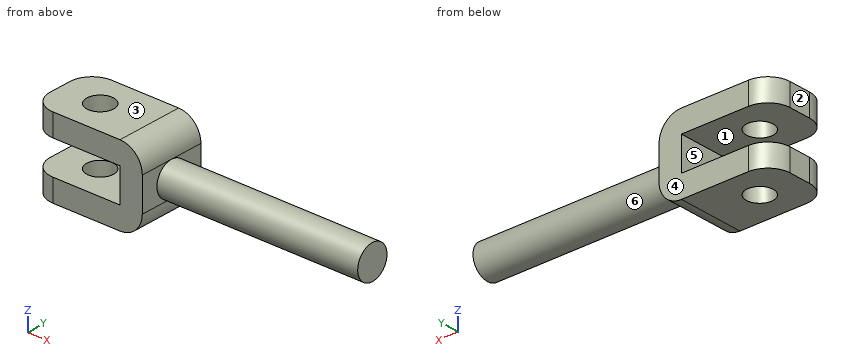
```python
from build123d import *

# Parameters (mm, degrees)
SKETCH1_R                = 0.75
BOSS_EXTRUDE1_DEPTH      = 10
BOSS_EXTRUDE2_DEPTH      = 1.5
BOSS_EXTRUDE2_DEPTH_BACK = 1.5
FILLET1_R                = 1
SKETCH3_R                = 0.6
CUT_EXTRUDE1_DEPTH       = 5


with BuildPart() as part:
    # Sketch1 → Boss-Extrude1 (new body)
    with BuildSketch(Plane(origin=(0, 0, 0), x_dir=(0, 0, -1), z_dir=(1, 0, 0))):
        Circle(SKETCH1_R)
    extrude(amount=BOSS_EXTRUDE1_DEPTH)

    # Sketch2 → Boss-Extrude2 (add, two sides: drawn at the far end of the back side and taken through both)
    with BuildSketch(Plane(origin=(0, 0, 0), x_dir=(1, 0, 0), z_dir=(0, 1, 0)).offset(-BOSS_EXTRUDE2_DEPTH_BACK)):
        Polygon((1, 1.75), (1, -1.75), (-4, -1.75), (-4, -0.75), (0, -0.75), (0, 0.75), (-4, 0.75), (-4, 1.75), align=None)
    extrude(amount=BOSS_EXTRUDE2_DEPTH + BOSS_EXTRUDE2_DEPTH_BACK)

    # Fillet1
    fillet1_edges = [part.edges().sort_by_distance(p)[0] for p in [
        (-4, 1.5, 1.25),
        (-4, 1.5, -1.25),
        (-4, -1.5, -1.25),
        (1, 0, -1.75),
        (1, 0, 1.75),
        (-4, -1.5, 1.25),
    ]]
    fillet(fillet1_edges, radius=FILLET1_R - 0.0001)  # a hair under: the kernel refuses the full size

    # Sketch3 → Cut-Extrude1 (cut)
    with BuildSketch(Plane(origin=(0, 0, -1.75), x_dir=(-1, 0, 0), z_dir=(0, 0, -1))):
        with Locations((2.2, 0)):
            Circle(SKETCH3_R)
    extrude(amount=-CUT_EXTRUDE1_DEPTH, mode=Mode.SUBTRACT)


solid = part.part
```
Geometry check sheet. Reference: the model listing, model coordinates, mm. Face numbers are marked on the shaded views. A direction names the side the tool comes from. Coordinates: 2 decimals unless noted, no trailing zeros. Order: outer loops, then holes, each group sorted by start corner. A loop starts at its lowest first (then second) coordinate and runs counter-clockwise, first axis right, second up. Notation, with made-up numbers: M 50,87.5 L 94,87.5 A12 ccw 94,107.5 Z; hole C -39,12 d6. An arc over 180 degrees is marked long. One line per question, with ' | ' between items. Start each with the question number.
Item 1: Gauge pin test, flat ends, axial feed: pin 1 (0.8 mm diameter, centred on y = 0.5, z = 0, fed in from -X); pin 2 (1.5 mm diameter, centred on x = 2, y = -1, fed in from +Z). Record the tip position at first contact, or that the pin passes through.
Item 2: Cross-section at B-B on z = 0. Enter the section's corners in (x, y), then the cut area to 3 significant figures.
Item 3: Cross-section at A-A on x = -2.2. Enter the section's corners in (y, z).
Item 4: Set-up check for the marked faces 4, 5 and 6: record each of +Z, -Z, +X, -X, +Y, -Y from which the full face is reachable in a straight line by a thin tool's end or side.
Item 5: Draft check along Z on the marked faces 1, 2 and 3. Enter one of: pulls with the +Z half, pulls with the -Z half, needs draft (parallel to the pull), parting line crosses it, or undercut.
Item 6: Cross-section at D-D on x = 8. Enter the section's corners in (y, z), then the cut area to 3 significant figures.
Item 7: Material ranges on L1, parallel to Z at x = -0.5, y = -0.2; L2, parallel to Y at x = -2.2, z = -1.15; L3, parallel to X at y = 0.75, z = 0.55, recorded low to high. Write a range as [from, to].
Item 8: Cross-section at C-C on z = -1. Enter the section's corners in (x, y), then the cut area to 3 significant figures.
Findings:
1) pin 1: stops at x = 0 | pin 2: stops at z = 0.71
2) outline: M 0,-1.5 L 1,-1.5 L 1,-0.75 L 10,-0.75 L 10,0.75 L 1,0.75 L 1,1.5 L 0,1.5 Z | area: 16.5 mm²
3) outline: M -1.5,-1.75 L -0.6,-1.75 L -0.6,-0.75 L -1.5,-0.75 Z; M -1.5,0.75 L -0.6,0.75 L -0.6,1.75 L -1.5,1.75 Z; M 0.6,-1.75 L 1.5,-1.75 L 1.5,-0.75 L 0.6,-0.75 Z; M 0.6,0.75 L 1.5,0.75 L 1.5,1.75 L 0.6,1.75 Z
4) face 4: +Z, -Z, +X, -X, +Y | face 5: -X, +Y, -Y | face 6: +X
5) face 1: undercut | face 2: needs draft | face 3: pulls with the +Z half
6) outline: C 0,0 d1.5 | area: 1.77 mm²
7) L1: z = [-1.75, -0.75], [0.75, 1.75] | L2: y = [-1.5, -0.6], [0.6, 1.5] | L3: x = [0, 1]
8) outline: M -4,-0.5 A1 ccw -3,-1.5 L 0.97,-1.5 L 0.97,1.5 L -3,1.5 A1 ccw -4,0.5 Z; hole C -2.2,0 d1.2 | area: 13.3 mm²
